```python
from build123d import *

# Parameters (mm, degrees)
SKETCH1_W           = 300
SKETCH1_H           = 150
BOSS_EXTRUDE1_DEPTH = 5
BOSS_EXTRUDE2_DEPTH = 147


with BuildPart() as part:
    # Sketch1 → Boss-Extrude1 (new body)
    with BuildSketch(Plane(origin=(0, 0, 0), x_dir=(1, 0, 0), z_dir=(0, 1, 0))):
        Rectangle(SKETCH1_W, SKETCH1_H)
    extrude(amount=BOSS_EXTRUDE1_DEPTH)

    # Sketch2 → Boss-Extrude2 (add)
    with BuildSketch(Plane(origin=(0, 5, 0), x_dir=(1, 0, 0), z_dir=(0, 1, 0))):
        with BuildLine():
            Line((-45, 5), (45, 5))
            ThreePointArc((45, 5), (50, 0), (45, -5))
            Line((45, -5), (-45, -5))
            ThreePointArc((-45, -5), (-50, 0), (-45, 5))
        make_face()
    extrude(amount=BOSS_EXTRUDE2_DEPTH)


solid = part.part
```
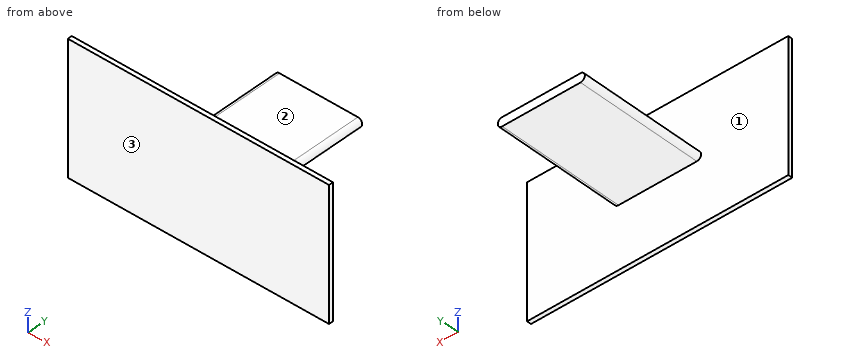
Geometry check sheet. Reference: the model listing, model coordinates, mm. Face numbers are marked on the shaded views. Give positions to 0.01 mm unless a question says otherwise; leave off trailing zeros. Loops run counter-clockwise (first coordinate to the right, second up) from the corner with the lowest first, then second, coordinate; pieces in that order, holes last. Notation, with made-up numbers: M 26,-39.5 L 39,-39.5 A4 ccw 39,-32.5 Z; hole C 4,43.5 d8. An arc over 180 degrees is marked long. Write item = value, one per line. Start each with the question number.
1. Thickness scan on probe 1 along Y at (x, z) = (-111, -65.5); probe 2 along Z at (x, y) = (-0.5, 36.5). Record the ranges inside material, lowest first.
2. Section check B-B, the plane x = -31. Enter the section's corners in (y, z).
3. Section check A-A, the plane z = 0. Enter the section's corners in (x, y), plus the area to 3 significant figures.
4. Section check C-C, the plane y = 41.5. Enter the section's corners in (x, z).
5. Go/stop test with flat-tipped pins: P1, Ø1.5, axis at x = 9.5, y = 94, coming from the -Z side; P2, Ø6, axis at x = 27.5, y = 102.5, coming from the +Z side; P3, Ø1.5, axis at x = -95, z = 34, coming from the +Y side. Record where each tip stops, or that it passes through.
6. Section check D-D, the plane x = 105.5. Enter the section's corners in (y, z).
7. Draft check along Y on the marked faces 1, 2 and 3. Enter one of: +Y half, -Y half, draft (parallel to the pull), parting line (faces both ways), or undercut.
Values follow:
q1.probe_1 = 0 to 5
q1.probe_2 = -5 to 5
q2.outline = M 0,-75 L 5,-75 L 5,-5 L 152,-5 L 152,5 L 5,5 L 5,75 L 0,75 Z
q3.outline = M -150,0 L 150,0 L 150,5 L 50,5 L 50,152 L -50,152 L -50,5 L -150,5 Z
q3.area = 16,200 mm^2
q4.outline = M -45,-5 L 45,-5 A5 ccw 45,5 L -45,5 A5 ccw Z
q5.P1 = -5
q5.P2 = 5
q5.P3 = 5
q6.outline = M 0,-75 L 5,-75 L 5,75 L 0,75 Z
q7.face_1 = +Y half
q7.face_2 = draft
q7.face_3 = -Y half
